Model file for the job. Use its own axes, mm. Face numbers are marked on the shaded views. Coordinates: 2 decimals unless noted, no trailing zeros. Write each loop counter-clockwise with the first axis right and the second up, starting at its lowest first coordinate (ties: lowest second). Pieces come first, ordered by that corner, then holes. Notation, with made-up numbers: (49.25, 62.5) - (98.25, 62.5) arc R33 cw to (98.25, 98.5) - close; hole circle Ø11 at (-8, 12.25). An arc over 180 degrees is marked (long way). Put each result on its own line as item: value. Start each with the question number.
1. Drill centre lines: L1, parallel to Z at x = 0, y = 0.2; L2, parallel to Z at x = 1.25, y = 0.55; L3, parallel to X at y = 0.4, z = 8. Where is each one in solid material? Low to high. Write a range as from..to.
2. Saw through at B-B, the plane z = 0. Write the cut outline in (x, y).
3. Saw through at D-D, the plane y = 0.65. Write the cut outline in (x, z).
4. Saw through at A-A, the plane x = 0. Write the cut outline in (y, z), plus the area to 3 significant figures.
5. Saw through at C-C, the plane x = 9.5. Write the cut outline in (y, z).
6. Drop flat-ended pins along their axis: P1, Ø1.5, axis at x = 0, z = 4.5, coming from the +Y side; P2, Ø1.8, axis at x = 9.5, z = 0, coming from the -Y side; P3, Ø1, axis at x = 7.5, y = 1, coming from the -Z side. Give the stop position or say it passes through.
7. Pull direction Z, two halves, no side cores. Call the marked faces 1, 2, 3 and 4: released by +Z, released by -Z, zero draft, split by the parting line, or undercut.
```python
from build123d import *

# Parameters (mm, degrees)
F0_R     = 11.5
F2_DEPTH = 2
F3_T     = -0.3
F1_W     = 14
F1_H     = 6
F1_R     = 1
F1_R_2   = 1.5
F4_DEPTH = 2.001


with BuildPart() as f2:
    # F0 (on Front) → F2 (new body)
    with BuildSketch(Plane.XZ):
        Circle(F0_R)
    extrude(amount=-F2_DEPTH)

    # F3
    f3_openings = [f2.faces().sort_by_distance(p)[0] for p in [
        (0, 2, 0),
    ]]
    offset(amount=F3_T, openings=f3_openings)

    # F1 (on Front) → F4 (cut, through all)
    with BuildSketch(Plane.XZ):
        with Locations((0, 1.5)):
            Rectangle(F1_W, F1_H)
        with Locations((0, -7)):
            Circle(F1_R)
        with Locations((9.5, 0)):
            Circle(F1_R_2)
    extrude(amount=-F4_DEPTH, mode=Mode.SUBTRACT)


solid = f2.part
```
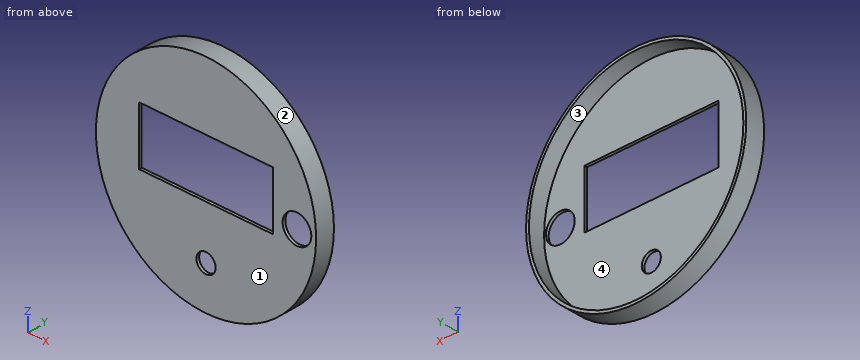
Final values:
1. L1: z = -11.5..-8, -6..-1.5, 4.5..11.5
1. L2: z = -11.43..-11.13, 11.13..11.43
1. L3: x = -8.26..-7.84, 7.84..8.26
2. outline: (-11.5, 0) - (-7, 0) - (-7, 0.3) - (-11.2, 0.3) - (-11.2, 2) - (-11.5, 2) - close; (7, 0) - (8, 0) - (8, 0.3) - (7, 0.3) - close; (11, 0) - (11.5, 0) - (11.5, 2) - (11.2, 2) - (11.2, 0.3) - (11, 0.3) - close
3. outline: circle Ø23 at (0, 0); hole circle Ø22.4 at (0, 0)
4. outline: (0, -11.5) - (2, -11.5) - (2, -11.2) - (0.3, -11.2) - (0.3, -8) - (0, -8) - close; (0, -6) - (0.3, -6) - (0.3, -1.5) - (0, -1.5) - close; (0, 4.5) - (0.3, 4.5) - (0.3, 11.2) - (2, 11.2) - (2, 11.5) - (0, 11.5) - close
4. area: 5.52 mm²
5. outline: (0, -6.48) - (2, -6.48) - (2, -5.93) - (0.3, -5.93) - (0.3, -1.5) - (0, -1.5) - close; (0, 1.5) - (0.3, 1.5) - (0.3, 5.93) - (2, 5.93) - (2, 6.48) - (0, 6.48) - close
6. P1: stops at y = 0.3
6. P2: passes through
6. P3: stops at z = -9.12
7. face 1: zero draft
7. face 2: split by the parting line
7. face 3: undercut
7. face 4: undercut
